```python
from build123d import *

# Parameters (mm, degrees)
SKETCH1_W               = 50
SKETCH1_H               = 275
BOSS_EXTRUDE1_DEPTH     = 7.5
BOSS_EXTRUDE2_DEPTH     = 7.5
SKETCH3_R               = 2.5
CUT_EXTRUDE1_DEPTH      = 280.609102141
CUT_EXTRUDE2_REACH      = 281.609
CUT_EXTRUDE3_DEPTH      = 280.609102141
CUT_EXTRUDE3_DEPTH_BACK = 280.609102141
SKETCH5_R               = 2.5


with BuildPart() as part:
    # Sketch1 → Boss-Extrude1 (new body)
    with BuildSketch(Plane.XY):
        with Locations((25, -137.5)):
            Rectangle(SKETCH1_W, SKETCH1_H)
    extrude(amount=BOSS_EXTRUDE1_DEPTH)

    # Sketch2 → Boss-Extrude2 (add)
    with BuildSketch(Plane.XY.offset(7.5)):
        Polygon((17.279404685, 0), (10, 20), (40, 20), (32.720595315, 0), align=None)
    extrude(amount=-BOSS_EXTRUDE2_DEPTH)

    # Sketch3 → Cut-Extrude1 (cut, through all)
    with BuildSketch(Plane.ZY):
        with Locations(Location((3.75, 15, 0), (0, 0, 270))):
            Circle(SKETCH3_R)
        with Locations(Location((3.75, 6, 0), (0, 0, 270))):
            Circle(SKETCH3_R)
    extrude(amount=-CUT_EXTRUDE1_DEPTH, mode=Mode.SUBTRACT)

    # Sketch4 → Cut-Extrude2 (cut, up to next)
    with BuildSketch(Plane.XY.offset(7.5), mode=Mode.PRIVATE) as cut_extrude2_sk1:
        Polygon((17.279404685, -275), (10, -255), (40, -255), (32.720595315, -275), align=None)
    cut_extrude2_tool1 = extrude(cut_extrude2_sk1.sketch, amount=-CUT_EXTRUDE2_REACH, mode=Mode.PRIVATE) & part.part
    add(cut_extrude2_tool1.solids().sort_by_distance((25, -263.93204, 7.5))[0], mode=Mode.SUBTRACT)

    # Sketch5 → Cut-Extrude3 (cut, two sides: drawn at the far end of the back side and taken through both)
    with BuildSketch(Plane.ZY.offset(-CUT_EXTRUDE3_DEPTH_BACK)):
        with Locations(Location((3.75, -269, 0), (0, 0, 270))):
            Circle(SKETCH5_R)
        with Locations(Location((3.75, -260, 0), (0, 0, 270))):
            Circle(SKETCH5_R)
    extrude(amount=CUT_EXTRUDE3_DEPTH + CUT_EXTRUDE3_DEPTH_BACK, mode=Mode.SUBTRACT)


solid = part.part
```
Verification items for the finished model (mm, model axes). A direction names the side the tool comes from. Coordinates: 2 decimals unless noted, no trailing zeros. Order: outer loops, then holes, each group sorted by start corner. A loop starts at its lowest first (then second) coordinate and runs counter-clockwise, first axis right, second up. Notation, with made-up numbers: (-28, 40.25) -> (8, 40.25) arc R13 ccw to (8, 59.25) -> close; hole circle Ø5 at (85, -11.5). An arc over 180 degrees is marked (long way). Answer as CSV lines item,"result". Start each with the question number.
1) Set-up check for faces 5 (the face through (25, 20, 4)), 6 (the face through (42.11, -271.31, 2.79)), 7 (the face through (41, 0, 4)), 8 (the face through (25, -255, 4)), 9 (the face through (9, 0, 4)): record each of +Z, -Z, +X, -X, +Y, -Y from which the full face is reachable in a straight line by a thin tool's end or side.
2) Material ranges on L1, parallel to Y at x = 30.5, z = 3.75; L2, parallel to Y at x = 44.5, z = 3.75; L3, parallel to Z at x = 5, y = -269, recorded low to high. Write a range as [from, to].
3) Release check for a two-part mould opening along Z. For faces 1 (the face through (0, -139, 4)), 2 (the face through (25, -125, 7.5)), 3 (the face through (43.72, -262.31, 2.79)), 4 (the face through (24.802, 17.498, 3.86)) record: released by +Z, released by -Z, zero draft, split by the parting line, or undercut.
4) Cross-section at A-A, the plane x = 4. Record the boundary of the cut face in (y, z).
5) Cross-section at B-B, the plane y = -269. Record the boundary of the cut face in (x, z).
6) Gauge pin test, flat ends, axial feed: pin 1 Ø3 at (y, z) = (-260, 3.75) entering from -X; pin 2 Ø1 at (x, z) = (41.5, 6) entering from +Y; pin 3 Ø6 at (x, y) = (32, -18) entering from -Z. Record the tip position at first contact, or that the pin passes through.
Conclusion:
1,face 5,"+Z, -Z, +X, -X, +Y"
1,face 6,"+X, -X"
1,face 7,"+Z, -Z, +X"
1,face 8,"+Z, -Z"
1,face 9,"+Z, -Z, -X"
2,L1,"y = [-255, 3.5], [8.5, 12.5], [17.5, 20]"
2,L2,"y = [-275, -271.5], [-266.5, -262.5], [-257.5, 0]"
2,L3,"z = [0, 1.25], [6.25, 7.5]"
3,face 1,"zero draft"
3,face 2,"released by +Z"
3,face 3,"undercut"
3,face 4,"undercut"
4,outline,"(-275, 0) -> (0, 0) -> (0, 7.5) -> (-275, 7.5) -> close; hole circle Ø5 at (-269, 3.75); hole circle Ø5 at (-260, 3.75)"
5,outline,"(0, 0) -> (15.1, 0) -> (15.1, 1.25) -> (0, 1.25) -> close; (0, 6.25) -> (15.1, 6.25) -> (15.1, 7.5) -> (0, 7.5) -> close; (34.9, 0) -> (50, 0) -> (50, 1.25) -> (34.9, 1.25) -> close; (34.9, 6.25) -> (50, 6.25) -> (50, 7.5) -> (34.9, 7.5) -> close"
6,pin 1,"passes through"
6,pin 2,"stops at y = 0"
6,pin 3,"stops at z = 0"
